from build123d import *

# Parameters (mm, degrees)
F1_DEPTH = 20
F2_W     = 20
F2_H     = 20
F3_DEPTH = 26.001
F5_DEPTH = 40.001
F7_DEPTH = 40.001


with BuildPart() as f1:
    # F0 (on Top) → F1 (new body, symmetric)
    with BuildSketch(Plane.XY):
        Polygon((0, 26), (0, 0), (10, 0), (10, 13), (50, 13), (50, 39), (40, 39), (40, 26), align=None)
    extrude(amount=F1_DEPTH, both=True)

    # F2 (on face) → F3 (cut, through all)
    with BuildSketch(Plane.XZ.offset(-13)):
        with Locations((40, 0)):
            Rectangle(F2_W, F2_H)
    extrude(amount=-F3_DEPTH, mode=Mode.SUBTRACT)

    # F4 (on face) → F5 (cut, through all)
    with BuildSketch(Plane.XY.offset(20)):
        Polygon((0, 0), (10, 0), (0, 13), align=None)
    extrude(amount=-F5_DEPTH, mode=Mode.SUBTRACT)

    # F6 (on face) → F7 (cut, through all)
    with BuildSketch(Plane.XY.offset(20)):
        Polygon((0, 13), (10, 26), (0, 26), align=None)
    extrude(amount=-F7_DEPTH, mode=Mode.SUBTRACT)


solid = f1.part
Input: part model. Units: mm. Frame: model coordinates. A direction names the side the tool comes from. Coordinates: 2 decimals unless noted, no trailing zeros. Loops run counter-clockwise (first coordinate to the right, second up) from the corner with the lowest first, then second, coordinate; pieces in that order, holes last. Notation, with made-up numbers: (49.5, 3.25) - (92.5, 3.25) arc R19 cw to (92.5, 10.25) - close; hole circle Ø8 at (28.5, 34). An arc over 180 degrees is marked (long way). Answer in a Markdown table with one row per item. Add a question column.
Item 1: Access query for faces 1 (the flat face through (10, 6, 0)), 2 (the flat face through (22, 26, 0)), 3 (the flat face through (30, 19, 0)). Directions: +Z, -Z, +X, -X, +Y, -Y. A direction counts if a zero-diameter tool reaches every point of the face in a straight line with its end or side. Return the directions, or none.
Item 2: Section query A-A on x = 41. Return the cut outline in (y, z).
Item 3: Line query: line 1 along Z through (x, y) = (33.5, 23.5); line 2 along X through (y, z) = (29, 18); line 3 along Y through (x, z) = (28.5, -4). Output: solid intervals per line, ascending. Write a range as [from, to].
Item 4: Section query C-C on z = -11. Return the cut outline in (x, y), then the cut area to 3 significant figures.
Item 5: Contact query for flat-ended pins moving along their axis: P1, Ø11, axis at y = 32.5, z = 13, coming from the -X side; P2, Ø12, axis at x = 13.5, z = 1.5, coming from the +Y side; P3, Ø1.5, axis at y = 24.5, z = 15, coming from the -X side; P4, Ø8, axis at y = 11, z = -8.5, coming from the +X side. Output: stop coordinate, or through.
Item 6: Section query D-D on y = 21.5. Return the cut outline in (x, z).
Item 7: Section query B-B on y = 27.5. Return the cut outline in (x, z), then the cut area to 3 significant figures.
Recorded:
| question | item | result |
|---|---|---|
| 1 | face 1 | +Z, -Z, +X, -Y |
| 1 | face 2 | +Z, -Z, -X, +Y |
| 1 | face 3 | +X, +Y, -Y |
| 2 | outline | (13, -20) - (39, -20) - (39, -10) - (13, -10) - close; (13, 10) - (39, 10) - (39, 20) - (13, 20) - close |
| 3 | line 1 | [-20, -10], [10, 20] |
| 3 | line 2 | [40, 50] |
| 3 | line 3 | [13, 26] |
| 4 | outline | (0, 13) - (10, 0) - (10, 13) - (50, 13) - (50, 39) - (40, 39) - (40, 26) - (10, 26) - close |
| 4 | area | 780 mm^2 |
| 5 | P1 | x = 40 |
| 5 | P2 | y = 26 |
| 5 | P3 | x = 8.27 |
| 5 | P4 | x = 50 |
| 6 | outline | (6.54, -20) - (50, -20) - (50, -10) - (30, -10) - (30, 10) - (50, 10) - (50, 20) - (6.54, 20) - close |
| 7 | outline | (40, -20) - (50, -20) - (50, -10) - (40, -10) - close; (40, 10) - (50, 10) - (50, 20) - (40, 20) - close |
| 7 | area | 200 mm^2 |
